Input: part model. Units: mm. Frame: model coordinates. A direction names the side the tool comes from. Coordinates: 2 decimals unless noted, no trailing zeros. Write each loop counter-clockwise with the first axis right and the second up, starting at its lowest first coordinate (ties: lowest second). Pieces come first, ordered by that corner, then holes. Notation, with made-up numbers: (-33, 65) - (-18, 65) arc R20 cw to (-18, 94) - close; hole circle Ø6 at (22, 74.5). An arc over 180 degrees is marked (long way). Use CSV: the item, a comma, the result in double quotes.
```python
from build123d import *

# Parameters (mm, degrees)
SKETCH_1_W          = 53.8
SKETCH_1_H          = 28.4
EXTRUDE_1_DEPTH     = 1
EXTRUDE_2_DEPTH     = 8
SKETCH_4_W          = 23.427026947
SKETCH_4_H          = 24.4
SKETCH_4_W_2        = 24.872973053
CUT_EXTRUDE_1_DEPTH = 62.497967446


with BuildPart() as part:
    # 草图1 → 凸台-拉伸1 (new body)
    with BuildSketch(Plane(origin=(0, 0, 0), x_dir=(1, 0, 0), z_dir=(0, 1, 0))):
        with Locations((26.9, -14.2)):
            Rectangle(SKETCH_1_W, SKETCH_1_H)
    extrude(amount=EXTRUDE_1_DEPTH)

    # 草图2 → 凸台-拉伸2 (add)
    with BuildSketch(Plane(origin=(0, 1, 0), x_dir=(1, 0, 0), z_dir=(0, 1, 0))):
        Polygon((53.8, -28.4), (53.621994937, -28.4), (50.621994937, -28.4), (50.621994937, -27.4), (52.8, -27.4), (52.8, -24.4), (53.8, -24.4), align=None)
        Polygon((53.8, 0), (52.8, 0), (49.8, 0), (49.8, -1), (52.8, -1), (52.8, -4), (53.8, -4), align=None)
        Polygon((0, -27.4), (0, -24.4), (1, -24.4), (1, -27.4), (4, -27.4), (4, -28.4), (0, -28.4), align=None)
        Polygon((0, 0), (4, 0), (4, -1), (1, -1), (1, -4), (0, -4), (0, -1), align=None)
    extrude(amount=EXTRUDE_2_DEPTH)

    # 草图4 → 切除-拉伸1 (cut, through all)
    with BuildSketch(Plane.XZ):
        with Locations((40.086486527, 14.2)):
            Rectangle(SKETCH_4_W, SKETCH_4_H)
        with Locations((14.436486527, 14.2)):
            Rectangle(SKETCH_4_W_2, SKETCH_4_H)
    extrude(amount=-CUT_EXTRUDE_1_DEPTH, mode=Mode.SUBTRACT)


solid = part.part
```
(1) Cut plane A-A on y = 5. Return loops of the section in (x, z).
Check values:
outline,"(0, 0) - (4, 0) - (4, 1) - (1, 1) - (1, 4) - (0, 4) - close; (0, 24.4) - (1, 24.4) - (1, 27.4) - (4, 27.4) - (4, 28.4) - (0, 28.4) - close; (49.8, 0) - (53.8, 0) - (53.8, 4) - (52.8, 4) - (52.8, 1) - (49.8, 1) - close; (50.62, 27.4) - (52.8, 27.4) - (52.8, 24.4) - (53.8, 24.4) - (53.8, 28.4) - (50.62, 28.4) - close"
(2) Draft query along X for faces 6 (the flat face through (53, 5, 4)), 7 (the flat face through (28.373, 0.5, 14)). Return one class per face: pulls with the +X half, pulls with the -X half, needs draft (parallel to the pull), parting line crosses it, or undercut.
Check values:
face 6,"needs draft"
face 7,"undercut"
(3) Cut plane D-D on y = 0.5. Return loops of the section in (x, z).
Check values:
outline,"(0, 0) - (53.8, 0) - (53.8, 28.4) - (0, 28.4) - close; hole (2, 2) - (26.87, 2) - (26.87, 26.4) - (2, 26.4) - close; hole (28.37, 2) - (51.8, 2) - (51.8, 26.4) - (28.37, 26.4) - close"
(4) Cut plane C-C on z = 2.75. Return loops of the section in (x, y), and give its area (3 significant figures).
Check values:
outline,"(0, 0) - (2, 0) - (2, 1) - (1, 1) - (1, 9) - (0, 9) - close; (26.87, 0) - (28.37, 0) - (28.37, 1) - (26.87, 1) - close; (51.8, 0) - (53.8, 0) - (53.8, 9) - (52.8, 9) - (52.8, 1) - (51.8, 1) - close"
area,"21.5 mm^2"
(5) Ray query, probe 1 along Z at (x, y) = (24, 0.5); probe 2 along X at (y, z) = (5.5, 26.25); probe 3 along Z at (x, y) = (2, 6.25). Return the intervals inside material, ascending. Write a range as from..to.
Check values:
probe 1,"0..2, 26.4..28.4"
probe 2,"0..1, 52.8..53.8"
probe 3,"0..1, 27.4..28.4"
(6) Cut plane B-B on x = 29.5. Return loops of the section in (y, z).
Check values:
outline,"(0, 0) - (1, 0) - (1, 2) - (0, 2) - close; (0, 26.4) - (1, 26.4) - (1, 28.4) - (0, 28.4) - close"
(7) Reachability of faces 1 (the flat face through (50.622, 5, 28)), 2 (the flat face through (0.5, 4.9, 4)), 3 (the flat face through (2, 5, 27.4)), 4 (the flat face through (49.8, 4.9, 0.5)), 5 (the flat face through (26.873, 0.5, 14)) from +Z, -Z, +X, -X, +Y, -Y: full face, straight path, thin tool, end or side. Return the list, or none.
Check values:
face 1,"+Z, +Y"
face 2,"+X, -X, +Y"
face 3,"+Y"
face 4,"+Z, -Z, +Y"
face 5,"+Y, -Y"
(8) Pin query (flat end, axial travel): pin 1 Ø2 at (y, z) = (2.5, 17.5) entering from +X; pin 2 Ø8.5 at (x, z) = (31.5, 16.5) entering from +Y. Return the tip coordinate at first contact, or that it passes through.
Check values:
pin 1,"through"
pin 2,"y = 1"
